```python
from build123d import *

# Parameters (mm, degrees)
SKETCH2_W           = 10
SKETCH2_H           = 8
SKETCH2_R           = 1.6
BOSS_EXTRUDE1_DEPTH = 3
SKETCH3_W           = 10
SKETCH3_H           = 10
SKETCH3_R           = 1.6
BOSS_EXTRUDE2_DEPTH = 3
BOSS_EXTRUDE3_DEPTH = 1
FILLET1_R           = 1
FILLET2_R           = 1


with BuildPart() as part:
    # Sketch2 → Boss-Extrude1 (new body)
    with BuildSketch(Plane(origin=(0, 0, 0), x_dir=(1, 0, 0), z_dir=(0, 1, 0))):
        Rectangle(SKETCH2_W, SKETCH2_H)
        with Locations(Location((0, 0.5, 0), (0, 0, 270))):
            Circle(SKETCH2_R, mode=Mode.SUBTRACT)
    extrude(amount=BOSS_EXTRUDE1_DEPTH)

    # Sketch3 → Boss-Extrude2 (add)
    with BuildSketch(Plane.XY.offset(4)):
        with Locations((0, 5)):
            Rectangle(SKETCH3_W, SKETCH3_H)
        with Locations((0, 7)):
            Circle(SKETCH3_R, mode=Mode.SUBTRACT)
    extrude(amount=BOSS_EXTRUDE2_DEPTH)

    # Sketch4 → Boss-Extrude3 (add)
    with BuildSketch(Plane.ZY.offset(5)):
        Polygon((-4, 3), (4, 10), (7, 10), (7, 0), (-4, 0), align=None)
    boss_extrude3 = extrude(amount=BOSS_EXTRUDE3_DEPTH)

    # Mirror1: Boss-Extrude3 across plane
    add(boss_extrude3.mirror(Plane(origin=(0, 0, 0), x_dir=(0, 0, 1), z_dir=(1, 0, 0))))

    # Fillet1
    fillet1_edges = [part.edges().sort_by_distance(p)[0] for p in [
        (0, 3, 4),
    ]]
    fillet(fillet1_edges, radius=FILLET1_R)

    # Fillet2
    fillet2_edges = [part.edges().sort_by_distance(p)[0] for p in [
        (-5, 3, -0.5),
        (5, 3, -0.5),
        (5, 7, 4),
        (5, 3.292893219, 3.707106781),
        (-5, 7, 4),
        (-5, 3.292893219, 3.707106781),
    ]]
    fillet(fillet2_edges, radius=FILLET2_R)


solid = part.part
```
Could you check a few things on this model? Use its own coordinates, in mm. A direction names the side the tool comes from. Round coordinates to 2 decimals unless told otherwise and drop trailing zeros. Write each loop counter-clockwise with the first axis right and the second up, starting at its lowest first coordinate (ties: lowest second). Pieces come first, ordered by that corner, then holes. Notation, with made-up numbers: M 47,75 L 77,75 A11 cw 77,85 Z; hole C 47,72 d3. An arc over 180 degrees is marked long. Answer in a Markdown table with one row per item. Add a question column.
Q1. Will these pins go through, and if not, where does the flat tip stop? pin 1 Ø2 at (x, z) = (0.5, -2) entering from +Y; pin 2 Ø3 at (x, y) = (0.5, 8) entering from -Z.
Q2. If I drill on line 1 (X direction, y = 1.65, z = -0.5); line 2 (Y direction, x = 0, z = 5.25); line 3 (X direction, y = 5, z = -0.75), over which ranges is the centre line in solid material (lowest first)? Write a range as from..to.
Q3. If we mould it in two halves opening along X, with no side actions, what happens to faces 1 (the cylindrical face through (-0.35, 5.44, 5.48)), 2 (the flat face through (5.43, 6.45, -0.06)), 3 (the flat face through (6, 4, 3))? For each: +X half, -X half, draft (parallel to the pull), parting line (faces both ways), or undercut.
Q4. Imagine slicing it at D-D (x = -3.5). Please give me the cut outline in (y, z), then the cut area to 3 significant figures.
Q5. Imagine slicing it at C-C (y = 6.5). Please give me the cut outline in (x, z), then the cut area to 3 significant figures.
Q6. Imagine slicing it at B-B (z = -0.5). Please give me the cut outline in (x, y).
Q7. Imagine slicing it at A-A (x = 0). Please give me the cut outline in (y, z).
Q8. On a 3-axis mill with a long thin cutter (end or side, diameter ignored), from which of +Z, -Z, +X, -X, +Y, -Y can I reach the whole of each face in a straight line? I mean faces 4 (the flat face through (-5.43, 6.45, -0.06)), 5 (the cylindrical face through (-4.699, 3.285, -0.549)). Say none if no direction works.
Values:
| question | item | result |
|---|---|---|
| 1 | pin 1 | y = 3 |
| 1 | pin 2 | z = 4 |
| 2 | line 1 | -6..-1.6, 1.6..6 |
| 2 | line 2 | 0..5.4, 8.6..10 |
| 2 | line 3 | -6..-5, 5..6 |
| 3 | face 1 | undercut |
| 3 | face 2 | draft |
| 3 | face 3 | +X half |
| 4 | outline | M 0,-4 L 3,-4 L 3,3 A1 cw 4,4 L 10,4 L 10,7 L 0,7 Z |
| 4 | area | 54.2 mm^2 |
| 5 | outline | M -6,0 L -5,0 L -5,3 A1 cw -4,4 L -1.52,4 L -1.52,7 L -6,7 Z; M 1.52,4 L 4,4 A1 cw 5,3 L 5,0 L 6,0 L 6,7 L 1.52,7 Z |
| 5 | area | 35.3 mm^2 |
| 6 | outline | M -6,0 L -1.6,0 L -1.6,3 L -4,3 A1 cw -5,4 L -5,6.06 L -6,6.06 Z; M 1.6,0 L 6,0 L 6,6.06 L 5,6.06 L 5,4 A1 cw 4,3 L 1.6,3 Z |
| 7 | outline | M 0,-4 L 3,-4 L 3,-2.1 L 0,-2.1 Z; M 0,1.1 L 3,1.1 L 3,3 A1 cw 4,4 L 5.4,4 L 5.4,7 L 0,7 Z; M 8.6,4 L 10,4 L 10,7 L 8.6,7 Z |
| 8 | face 4 | -Z, +X, -X, +Y |
| 8 | face 5 | -Z, +Y |
